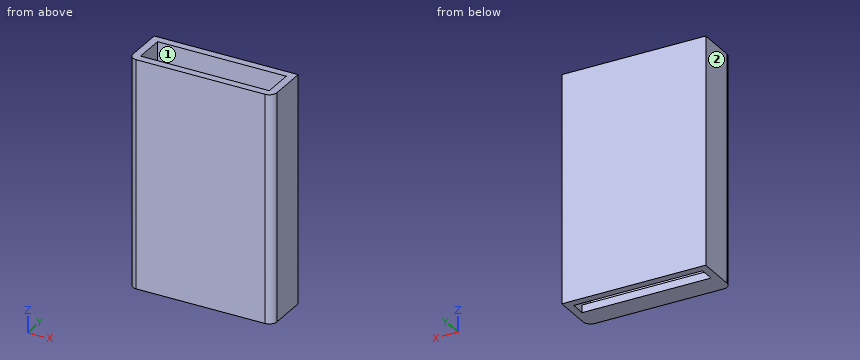
```python
from build123d import *

# Parameters (mm, degrees)
F0_W     = 24.13
F0_H     = 7.62
F0_W_2   = 21.59
F0_H_2   = 5.08
F1_DEPTH = 38.1
F2_W     = 22.86
F2_H     = 2.741368
F3_DEPTH = 1.27
F4_R     = 1.27


with BuildPart() as f1:
    # F0 (on Top) → F1 (new body)
    with BuildSketch(Plane.XY):
        Rectangle(F0_W, F0_H)
        Rectangle(F0_W_2, F0_H_2, mode=Mode.SUBTRACT)
    extrude(amount=F1_DEPTH)

    # F2 (on Top) → F3 (join)
    with BuildSketch(Plane.XY):
        with Locations((0.031765, -1.370684)):
            Rectangle(F2_W, F2_H)
    extrude(amount=F3_DEPTH)

    # F4
    f4_edges = [f1.edges().sort_by_distance(p)[0] for p in [
        (-12.065, -3.81, 19.05),
        (12.065, -3.81, 19.05),
    ]]
    fillet(f4_edges, radius=F4_R)


solid = f1.part
```
Design review of the part built by this model. Coordinates are the model's own, in mm. Face numbers are marked on the shaded views. A direction names the side the tool comes from. Give positions to 0.01 mm unless a question says otherwise; leave off trailing zeros. Loops run counter-clockwise (first coordinate to the right, second up) from the corner with the lowest first, then second, coordinate; pieces in that order, holes last. Notation, with made-up numbers: M 0.25,74.5 L 28.25,74.5 A26 ccw 28.25,101.5 Z; hole C 54,-4.5 d4. An arc over 180 degrees is marked long. Return JSON: item names as keys, results as strings. Group by question number.
Item 1: We need section B-B (y = 2). Give the boundary of the cut face in (x, z) (3 decimals), and give its area (3 significant figures).
Item 2: We need section D-D (y = -1.5). Give the boundary of the cut face in (x, z) (3 decimals).
Item 3: We need section C-C (x = 3.25). Give the boundary of the cut face in (y, z), and give its area (4 significant figures).
Item 4: Tool access review of the marked faces 1 and 2: name each direction out of +Z, -Z, +X, -X, +Y, -Y from which nothing blocks a thin tool from reaching the whole face with its end or side.
Item 5: Insertion check: pin 1 Ø2 at (x, y) = (-2, 0) entering from +Z. The pin has a flat end and moves straight along its axis. Give the tip position at first contact, or say it passes through.
Item 6: For probe 1 along X at (y, z) = (-2.5, 12) (3 decimals); probe 2 along Y at (x, z) = (5.75, 22); probe 3 along Z at (x, y) = (8, -0.5), list the stretches that pass through material, from the lowest coordinate up.
Item 7: We need section A-A (z = 21). Give the boundary of the cut face in (x, y) (3 decimals), and give its area (3 significant figures).
Output:
{
 "1": {"outline": "M -12.065,0 L -10.795,0 L -10.795,38.1 L -12.065,38.1 Z; M 10.795,0 L 12.065,0 L 12.065,38.1 L 10.795,38.1 Z", "area": "96.8 mm^2"},
 "2": {"outline": "M -12.065,0 L 12.065,0 L 12.065,38.1 L 10.795,38.1 L 10.795,1.27 L -10.795,1.27 L -10.795,38.1 L -12.065,38.1 Z"},
 "3": {"outline": "M -3.81,0 L 0,0 L 0,1.27 L -2.54,1.27 L -2.54,38.1 L -3.81,38.1 Z; M 2.54,0 L 3.81,0 L 3.81,38.1 L 2.54,38.1 Z", "area": "100.0 mm^2"},
 "4": {"face 1": "+Z, -Z", "face 2": "+Z, -Z, -X, +Y, -Y"},
 "5": {"pin 1": "stops at z = 1.27"},
 "6": {"probe 1": "x = -12.065 to -10.795, 10.795 to 12.065", "probe 2": "y = -3.81 to -2.54, 2.54 to 3.81", "probe 3": "z = 0 to 1.27"},
 "7": {"outline": "M -12.065,-2.54 A1.27 ccw -10.795,-3.81 L 10.795,-3.81 A1.27 ccw 12.065,-2.54 L 12.065,3.81 L -12.065,3.81 Z; hole M -10.795,-2.54 L 10.795,-2.54 L 10.795,2.54 L -10.795,2.54 Z", "area": "73.5 mm^2"}
}
